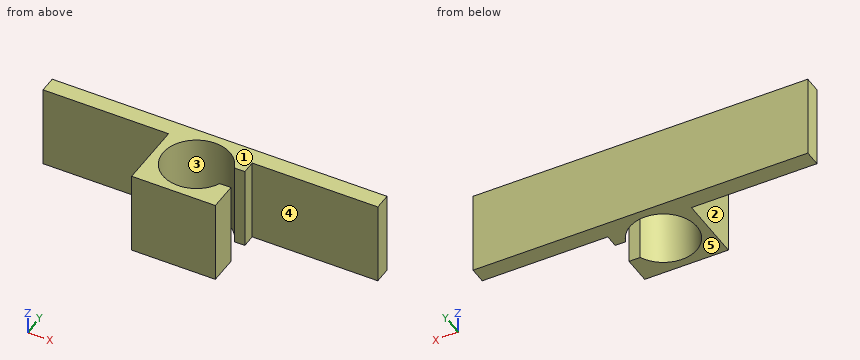
from build123d import *

# Parameters (mm, degrees)
F0_W     = 12.7
F0_H     = 12.7
F1_DEPTH = 12.7
F3_DEPTH = 38.1
F4_W     = 19.05
F4_H     = 12.7
F5_DEPTH = 2.54


with BuildPart() as f1:
    # F0 (on Front) → F1 (new body)
    with BuildSketch(Plane.XZ):
        with Locations((-32.274292, 11.265401)):
            Rectangle(F0_W, F0_H)
    extrude(amount=-F1_DEPTH)

    # F2 (on face) → F3 (cut)
    with BuildSketch(Plane.XY.offset(17.615401)):
        with BuildLine():
            Line((-25.924292, 8.11507), (-27.510793, 8.11507))
            ThreePointArc((-27.510793, 8.11507), (-37.352049, 6.500956), (-27.62406, 4.30507))
            Line((-27.62406, 4.30507), (-25.924292, 4.30507))
            Line((-25.924292, 4.30507), (-25.924292, 8.11507))
        make_face()
    extrude(amount=-F3_DEPTH, mode=Mode.SUBTRACT)

    # F4 (on face) → F5 (join)
    with BuildSketch(Plane(origin=(0, 12.7, 0), x_dir=(-1, 0, 0), z_dir=(0, 1, 0))):
        with Locations((48.149292, 11.265401)):
            Rectangle(F4_W, F4_H)
        with Locations((16.399292, 11.265401)):
            Rectangle(F4_W, F4_H)
    extrude(amount=-F5_DEPTH)


solid = f1.part
Input: part model. Units: mm. Frame: model coordinates. Face numbers are marked on the shaded views. A direction names the side the tool comes from. Coordinates: 2 decimals unless noted, no trailing zeros. Order: outer loops, then holes, each group sorted by start corner. A loop starts at its lowest first (then second) coordinate and runs counter-clockwise, first axis right, second up.
1. Access query for the marked faces 1 and 2. Directions: +Z, -Z, +X, -X, +Y, -Y. A direction counts if a zero-diameter tool reaches every point of the face in a straight line with its end or side. Return the directions, or none.
Checked values:
face 1: +Z, +X, -X, +Y, -Y
face 2: +Z, -Z, -X, -Y
2. Cut plane A-A, the plane x = -29. Return loops of the section in (y, z).
Checked values:
outline: (0, 4.92) - (2.47, 4.92) - (2.47, 17.62) - (0, 17.62) - close; (10.23, 4.92) - (12.7, 4.92) - (12.7, 17.62) - (10.23, 17.62) - close
3. Cut plane C-C, the plane y = 10.75. Return loops of the section in (x, z), plus the area to 3 significant figures.
Checked values:
outline: (-57.67, 4.92) - (-34.81, 4.92) - (-34.81, 17.62) - (-57.67, 17.62) - close; (-29.74, 4.92) - (-6.87, 4.92) - (-6.87, 17.62) - (-29.74, 17.62) - close
area: 581 mm2
4. Cut plane B-B, the plane z = 8. Return loops of the section in (x, y), plus the area to 3 significant figures.
Checked values:
outline: (-57.67, 10.16) - (-38.62, 10.16) - (-38.62, 0) - (-25.92, 0) - (-25.92, 4.31) - (-27.62, 4.31) arc R5.08 cw (long way) to (-27.51, 8.12) - (-25.92, 8.12) - (-25.92, 10.16) - (-6.87, 10.16) - (-6.87, 12.7) - (-57.67, 12.7) - close
area: 172 mm2
5. Contact query for flat-ended pins moving along their axis: P1, Ø1.5, axis at y = 1.5, z = 16, coming from the -X side; P2, Ø1.3, axis at x = -26.5, z = 12.5, coming from the -Y side; P3, Ø2, axis at y = 3, z = 13.5, coming from the +X side. Output: stop coordinate, or through.
Checked values:
P1: stops at x = -38.62
P2: stops at y = 0
P3: stops at x = -25.92
6. Ray query, line 1 along Y through (x, z) = (-42, 15.5); line 2 along X through (y, z) = (6.35, 10.5); line 3 along X through (y, z) = (8.25, 6). Return the intervals inside material, ascending.
Checked values:
line 1: y = 10.16 to 12.7
line 2: x = -38.62 to -37.35
line 3: x = -38.62 to -36.99, -27.56 to -25.92
7. Cut plane D-D, the plane y = 6.35. Return loops of the section in (x, z).
Checked values:
outline: (-38.62, 4.92) - (-37.35, 4.92) - (-37.35, 17.62) - (-38.62, 17.62) - close
8. Draft query along Y for the marked faces 3, 4 and 5. Return one class per face: +Y half, -Y half, draft (parallel to the pull), parting line (faces both ways), or undercut.
Checked values:
face 3: undercut
face 4: -Y half
face 5: draft
